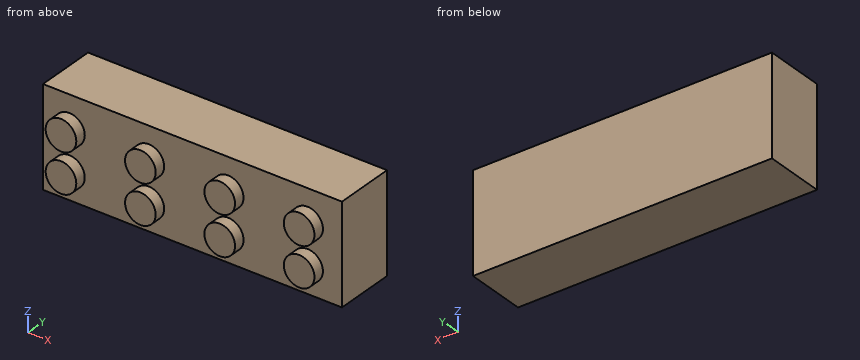
```python
from build123d import *

# Parameters (mm, degrees)
F0_W     = 47.8282
F0_H     = 15.9004
F1_DEPTH = 9.6012
F2_R     = 2.4511
F3_DEPTH = 1.8034


with BuildPart() as f1:
    # F0 (on Front) → F1 (new body)
    with BuildSketch(Plane.XZ):
        with Locations((-23.9141, 7.9502)):
            Rectangle(F0_W, F0_H)
    extrude(amount=F1_DEPTH)

    # F2 (on face) → F3 (join)
    with BuildSketch(Plane.XZ.offset(9.6012)):
        with Locations((-5.4991, 10.659005)):
            Circle(F2_R)
        with Locations((-5.4991, 4.309005)):
            Circle(F2_R)
        with Locations((-18.1991, 10.659005)):
            Circle(F2_R)
        with Locations((-18.1991, 4.309005)):
            Circle(F2_R)
        with Locations((-30.8991, 10.659005)):
            Circle(F2_R)
        with Locations((-30.8991, 4.309005)):
            Circle(F2_R)
        with Locations((-43.5991, 10.659005)):
            Circle(F2_R)
        with Locations((-43.5991, 4.309005)):
            Circle(F2_R)
    extrude(amount=F3_DEPTH)


solid = f1.part
```
Check sheet for the modelled part. Datum: model origin and axes. Units: mm. Coordinates: 2 decimals unless noted, no trailing zeros. Write each loop counter-clockwise with the first axis right and the second up, starting at its lowest first coordinate (ties: lowest second). Pieces come first, ordered by that corner, then holes. Notation, with made-up numbers: (-19, -1) -> (17, -1) arc R22 cw to (17, 21) -> close; hole circle Ø6 at (36, -40). An arc over 180 degrees is marked (long way). Use a Markdown table: item, result.
1. Sectioned sample at A-A (x = -18.5). Enter the section's corners in (y, z), plus the area to 3 significant figures.
Reported:
| item | result |
|---|---|
| outline | (-11.4, 1.88) -> (-9.6, 1.88) -> (-9.6, 0) -> (0, 0) -> (0, 15.9) -> (-9.6, 15.9) -> (-9.6, 13.09) -> (-11.4, 13.09) -> (-11.4, 8.23) -> (-9.6, 8.23) -> (-9.6, 6.74) -> (-11.4, 6.74) -> close |
| area | 170 mm2 |
2. Sectioned sample at C-C (x = -42.5). Enter the section's corners in (y, z), plus the area to 3 significant figures.
Reported:
| item | result |
|---|---|
| outline | (-11.4, 2.12) -> (-9.6, 2.12) -> (-9.6, 0) -> (0, 0) -> (0, 15.9) -> (-9.6, 15.9) -> (-9.6, 12.85) -> (-11.4, 12.85) -> (-11.4, 8.47) -> (-9.6, 8.47) -> (-9.6, 6.5) -> (-11.4, 6.5) -> close |
| area | 168 mm2 |
3. Sectioned sample at D-D (z = 11.5). Enter the section's corners in (x, y), plus the area to 3 significant figures.
Reported:
| item | result |
|---|---|
| outline | (-47.83, -9.6) -> (-45.9, -9.6) -> (-45.9, -11.4) -> (-41.3, -11.4) -> (-41.3, -9.6) -> (-33.2, -9.6) -> (-33.2, -11.4) -> (-28.6, -11.4) -> (-28.6, -9.6) -> (-20.5, -9.6) -> (-20.5, -11.4) -> (-15.9, -11.4) -> (-15.9, -9.6) -> (-7.8, -9.6) -> (-7.8, -11.4) -> (-3.2, -11.4) -> (-3.2, -9.6) -> (0, -9.6) -> (0, 0) -> (-47.83, 0) -> close |
| area | 492 mm2 |
4. Scan lines: line 1 along Y through (x, z) = (-14.5, 7.5); line 2 along X through (y, z) = (-10.5, 11.5); line 3 along Z through (x, y) = (-19, -9.75). Record each from-to range of solid material in increasing order.
Reported:
| item | result |
|---|---|
| line 1 | y = -9.6 to 0 |
| line 2 | x = -45.9 to -41.3, -33.2 to -28.6, -20.5 to -15.9, -7.8 to -3.2 |
| line 3 | z = 1.99 to 6.63, 8.34 to 12.98 |
5. Sectioned sample at B-B (z = 9). Enter the section's corners in (x, y).
Reported:
| item | result |
|---|---|
| outline | (-47.83, -9.6) -> (-45.4, -9.6) -> (-45.4, -11.4) -> (-41.79, -11.4) -> (-41.79, -9.6) -> (-32.7, -9.6) -> (-32.7, -11.4) -> (-29.09, -11.4) -> (-29.09, -9.6) -> (-20, -9.6) -> (-20, -11.4) -> (-16.39, -11.4) -> (-16.39, -9.6) -> (-7.3, -9.6) -> (-7.3, -11.4) -> (-3.69, -11.4) -> (-3.69, -9.6) -> (0, -9.6) -> (0, 0) -> (-47.83, 0) -> close |
